Part model, mm, in its own coordinate system. A direction names the side the tool comes from. Round coordinates to 2 decimals unless told otherwise and drop trailing zeros. Order: outer loops, then holes, each group sorted by start corner. A loop starts at its lowest first (then second) coordinate and runs counter-clockwise, first axis right, second up. Notation, with made-up numbers: M 8,72.25 L 67,72.25 A12 ccw 67,85.25 Z; hole C 0,10.5 d7. An arc over 180 degrees is marked long. Write each question's results on one line, items separated by ' | '. Start each with the question number.
1. Probe L1, parallel to Z at x = 4.15, y = 0; L2, parallel to Y at x = 1.55, z = 0.9; L3, parallel to Y at x = 0.9, z = -0.8. List the from-to ranges inside material, lowest first. Write a range as [from, to].
2. Band-saw the part on A-A, the plane x = 4.55. List the corners of the cut face in (y, z).
3. Drop flat-ended pins along their axis: pin 1 Ø1.2 at (x, y) = (1, 0) entering from -Z; pin 2 Ø1.5 at (x, y) = (2, 0) entering from -Z; pin 3 Ø1 at (x, z) = (5, -0.5) entering from +Y. Give the stop position or say it passes through.
4. Which spindle directions (+Z, -Z, +X, -X, +Y, -Y) get a long thin tool onto all of the face, cutting with end or side? Do faces 4 (the face through (0, 1, -1)), 5 (the face through (0.5, 0, 1.2)). Say none if no direction does.
5. Two-plate mould, pull along Y, no slides. Class faces 1 (the face through (0.5, 0, -1.2)), 2 (the face through (3.53, -1.5, 0.07)), 3 (the face through (6, 0, 0)): +Y half, -Y half, draft (parallel to the pull), parting line (faces both ways), or undercut.
Autodesk Inventor part; units mm, degrees
ref_plane "screw_XY" through (5.5, 0, 0) normal (1, 0, 0) x (0, 0, -1)
ref_plane "screw_YZ" through (5.5, 0, 0) normal (0, 0, -1) x (0, 1, 0)
ref_plane "screw_ZX" through (5.5, 0, 0) normal (0, 1, 0) x (1, 0, 0)
sketch "Sketch_8" plane through (0, 0, 0) normal (0, 0, 1) x (1, 0, 0)
  line L0 (6, 0) -> (0, 0)
  line L1 (0, 0) -> (0, 2.8)
  line L2 (0, 2.8) -> (1.3, 1.5)
  line L3 (1.3, 1.5) -> (5.6935, 1.5)
  line L4 (5.6935, 1.5) -> (6, 1.1935)
  line L5 (6, 1.1935) -> (6, 0)
  line L6 (6, 0) -> (0, 0)
revolve "Revolution1" add sketch "Sketch_8" angle 360 about axis through (6, 0, 0) along (1, 0, 0)
thread "Thread1"
sketch "Sketch_9" plane through (0, 0, 0) normal (0, 1, 0) x (-1, 0, 0)
  line L0 (-1.4215, 0) -> (0, 0)
  line L1 (0, 0) -> (0, -1.2)
  line L2 (0, -1.2) -> (-1.1, -1.2)
  line L3 (-1.1, -1.2) -> (-1.4215, 0)
  line L4 (-1.4215, 0) -> (0, 0)
revolve "Revolution2" cut sketch "Sketch_9" angle 360 about axis through (1.4215, 0, 0) along (1, 0, 0)
sketch "Sketch_10" plane through (0, 0, 0) normal (1, 0, 0) x (0, 1, 0)
  line L0 (0.6928, 1.2) -> (-0.6928, 1.2)
  line L1 (-0.6928, 1.2) -> (-1.3856, 0)
  line L2 (-1.3856, 0) -> (-0.6928, -1.2)
  line L3 (-0.6928, -1.2) -> (0.6928, -1.2)
  line L4 (0.6928, -1.2) -> (1.3856, 0)
  line L5 (1.3856, 0) -> (0.6928, 1.2)
extrude "Extrusion1" cut sketch "Sketch_10" along normal blind 1.1
ref_plane "screw_XY" through (5.5, 0, 0) normal (1, 0, 0) x (0, 0, -1)
ref_plane "screw_YZ" through (5.5, 0, 0) normal (0, 0, -1) x (0, 1, 0)
ref_plane "screw_ZX" through (5.5, 0, 0) normal (0, 1, 0) x (1, 0, 0)
ref_plane "to_nut_XY" through (6, 0, 0) normal (1, 0, 0) x (0, 0, -1)
ref_plane "to_nut_YZ" through (6, 0, 0) normal (0, 0, -1) x (0, 1, 0)
ref_plane "to_nut_ZX" through (6, 0, 0) normal (0, 1, 0) x (1, 0, 0)
ref_plane "xx_XY" through (0.8, 0, 0) normal (1, 0, 0) x (0, 0, -1)
ref_plane "xx_YZ" through (0.8, 0, 0) normal (0, 0, -1) x (0, 1, 0)
ref_plane "xx_ZX" through (0.8, 0, 0) normal (0, 1, 0) x (1, 0, 0)
properties part number "FB3-6s"
Solution:
1) L1: [-1.5, 1.5] | L2: [-1.2, 1.2] | L3: [-1.72, -0.92], [0.92, 1.72]
2) outline: C 0,0 d3
3) pin 1: z = -2.4 | pin 2: z = -1.55 | pin 3: y = 1.5
4) face 4: +Z, -Z, -X, +Y, -Y | face 5: -X
5) face 1: undercut | face 2: parting line | face 3: draft
